```python
from build123d import *

# Parameters (mm, degrees)
SKETCH1_W           = 20
SKETCH1_H           = 20
BOSS_EXTRUDE1_DEPTH = 2.5
FILLET1_R           = 5
SKETCH2_R           = 1.5
CUT_EXTRUDE1_DEPTH  = 10
CUT_EXTRUDE2_DEPTH  = 1.5
SKETCH4_W           = 7
SKETCH4_H           = 1
BOSS_EXTRUDE2_DEPTH = 2
FILLET2_R           = 1


with BuildPart() as part:
    # Sketch1 → Boss-Extrude1 (new body)
    with BuildSketch(Plane(origin=(0, 0, 0), x_dir=(1, 0, 0), z_dir=(0, 1, 0))):
        Rectangle(SKETCH1_W, SKETCH1_H)
    extrude(amount=BOSS_EXTRUDE1_DEPTH)

    # Fillet1
    fillet1_edges = [part.edges().sort_by_distance(p)[0] for p in [
        (10, 1.25, 10),
        (-10, 1.25, 10),
        (-10, 1.25, -10),
        (10, 1.25, -10),
    ]]
    fillet(fillet1_edges, radius=FILLET1_R)

    # Sketch2 → Cut-Extrude1 (cut)
    with BuildSketch(Plane(origin=(0, 2.5, 0), x_dir=(1, 0, 0), z_dir=(0, 1, 0))):
        with Locations(Location((5.656854249, -5.656854249, 0), (0, 0, 270))):
            Circle(SKETCH2_R)
        with Locations(Location((-5.656854249, 5.656854249, 0), (0, 0, 270))):
            Circle(SKETCH2_R)
    extrude(amount=-CUT_EXTRUDE1_DEPTH, mode=Mode.SUBTRACT)

    # Sketch3 → Cut-Extrude2 (cut)
    with BuildSketch(Plane(origin=(0, 2.5, 0), x_dir=(1, 0, 0), z_dir=(0, 1, 0))):
        with BuildLine():
            Line((5, 9), (-5, 9))
            ThreePointArc((-5, 9), (-7.828427125, 7.828427125), (-9, 5))
            Line((-9, 5), (-9, -5))
            ThreePointArc((-9, -5), (-7.828427125, -7.828427125), (-5, -9))
            Line((-5, -9), (5, -9))
            ThreePointArc((5, -9), (7.828427125, -7.828427125), (9, -5))
            Line((9, -5), (9, 5))
            ThreePointArc((9, 5), (7.828427125, 7.828427125), (5, 9))
        make_face()
    extrude(amount=-CUT_EXTRUDE2_DEPTH, mode=Mode.SUBTRACT)

    # Sketch4 → Boss-Extrude2 (add)
    with BuildSketch(Plane(origin=(0, 2.5, 0), x_dir=(1, 0, 0), z_dir=(0, 1, 0))):
        with Locations((0, 9.5)):
            Rectangle(SKETCH4_W, SKETCH4_H)
        with Locations((0, -9.5)):
            Rectangle(SKETCH4_W, SKETCH4_H)
    extrude(amount=BOSS_EXTRUDE2_DEPTH)

    # Fillet2
    fillet2_edges = [part.edges().sort_by_distance(p)[0] for p in [
        (-3.5, 4.5, -9.5),
        (3.5, 4.5, -9.5),
        (-3.5, 4.5, 9.5),
        (3.5, 4.5, 9.5),
    ]]
    fillet(fillet2_edges, radius=FILLET2_R)


solid = part.part
```
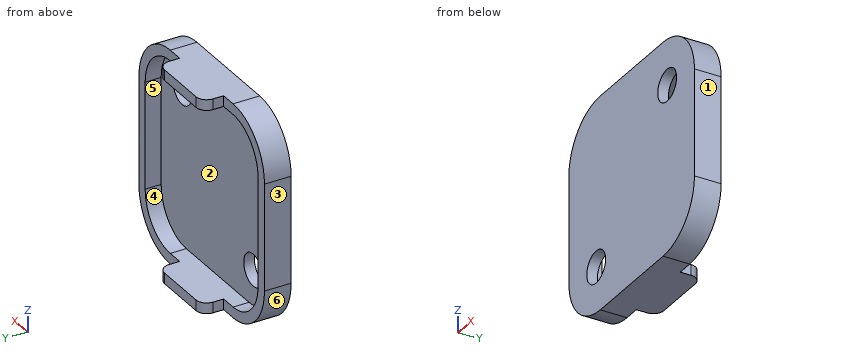
Here's how the part is built. I have some questions about the finished solid (model axes, mm). Face numbers are marked on the shaded views. A direction names the side the tool comes from. Give positions to 0.01 mm unless a question says otherwise; leave off trailing zeros. Loops run counter-clockwise (first coordinate to the right, second up) from the corner with the lowest first, then second, coordinate; pieces in that order, holes last. Notation, with made-up numbers: M -2,29.25 L 48,29.25 A16 ccw 48,38.25 Z; hole C 39.5,76.25 d1. An arc over 180 degrees is marked long. Put each result on its own line as item: value. Start each with the question number.
(1) I need wall thicknesses on line 1 along Z through (x, y) = (0.5, 4.15); line 2 along Y through (x, z) = (4.5, -1). Which ranges of each line are inside material? Lowest first, please. Write a range as [from, to].
(2) I want a section at A-A on z = 1. Please give me the cut outline in (x, y), then the cut area to 3 significant figures.
(3) If we mould it in two halves opening along Z, with no side actions, what happens to the marked faces 3, 4, 5 and 6? For each: +Z half, -Z half, draft (parallel to the pull), parting line (faces both ways), or undercut.
(4) I want a section at C-C on y = 3.75. Please give me the cut outline in (x, z), then the cut area to 3 significant figures.
(5) I want a section at B-B on y = 1.45. Please give me the cut outline in (x, z).
(6) For the marked faces 1 and 2, which set-ups out of +Z, -Z, +X, -X, +Y, -Y let a thin tool reach every point of the face, with its end or its side?
(7) I want a section at D-D on x = 1.75. Please give me the cut outline in (y, z).
(8) Will these pins go through, and if not, where does the flat tip stop? pin 1 Ø2 at (x, y) = (-7, 0.5) entering from -Z; pin 2 Ø5 at (x, z) = (5, -3) entering from +Y; pin 3 Ø0.8 at (y, z) = (3, 9.5) entering from -X.
Answer block:
1. line 1: [-10, -9], [9, 10]
1. line 2: [0, 1]
2. outline: M -10,0 L 10,0 L 10,2.5 L 9,2.5 L 9,1 L -9,1 L -9,2.5 L -10,2.5 Z
2. area: 23.0 mm^2
3. face 3: draft
3. face 4: undercut
3. face 5: undercut
3. face 6: -Z half
4. outline: M -3.47,-10 L 3.47,-10 L 3.47,-9 L -3.47,-9 Z; M -3.47,9 L 3.47,9 L 3.47,10 L -3.47,10 Z
4. area: 13.9 mm^2
5. outline: M -10,-5 A5 ccw -5,-10 L 5,-10 A5 ccw 10,-5 L 10,5 A5 ccw 5,10 L -5,10 A5 ccw -10,5 Z; hole M -9,-5 A4 ccw -5,-9 L 5,-9 A4 ccw 9,-5 L 9,5 A4 ccw 5,9 L -5,9 A4 ccw -9,5 Z
6. face 1: +Z, -Z, +X, +Y, -Y
6. face 2: +Y
7. outline: M 0,-10 L 4.5,-10 L 4.5,-9 L 1,-9 L 1,9 L 4.5,9 L 4.5,10 L 0,10 Z
8. pin 1: z = -9.9
8. pin 2: y = 1
8. pin 3: x = -3.5
